Model file for the job. Use its own axes, mm. Round coordinates to 2 decimals unless told otherwise and drop trailing zeros. Order: outer loops, then holes, each group sorted by start corner. A loop starts at its lowest first (then second) coordinate and runs counter-clockwise, first axis right, second up. Notation, with made-up numbers: (53.5, 16.5) - (71.5, 16.5) arc R23 cw to (71.5, 40.5) - close; hole circle Ø4 at (-4.5, 36.5). An arc over 180 degrees is marked (long way). Use one line per item in the form item = value.
from build123d import *

# Parameters (mm, degrees)
SKETCH1_W               = 210
SKETCH1_H               = 110
TOP_DEPTH               = 5
SKETCH2_W               = 200
SKETCH2_H               = 100
BOTTOM_DEPTH            = 6
HOLE_REACH              = 120.684
SKETCH4_R               = 1.5
HOLE_PATTERN_COUNT      = 2
HOLE_PATTERN_PITCH      = 105
HOLE_PATTERN_COUNT_DIR2 = 2
HOLE_PATTERN_PITCH_DIR2 = 205


with BuildPart() as part:
    # Sketch1 → Top (new body)
    with BuildSketch(Plane(origin=(0, 0, 0), x_dir=(1, 0, 0), z_dir=(0, 1, 0))):
        Rectangle(SKETCH1_W, SKETCH1_H)
    extrude(amount=TOP_DEPTH)

    # Sketch2 → Bottom (add)
    with BuildSketch(Plane(origin=(0, 5, 0), x_dir=(1, 0, 0), z_dir=(0, 1, 0))):
        Rectangle(SKETCH2_W, SKETCH2_H)
    extrude(amount=BOTTOM_DEPTH)

    # Sketch4 → Hole (cut, up to next)
    with BuildSketch(Plane(origin=(0, 5, 0), x_dir=(1, 0, 0), z_dir=(0, 1, 0)), mode=Mode.PRIVATE) as hole_sk1:
        with Locations(Location((-102.5, -52.5, 0), (0, 0, 270))):
            Circle(SKETCH4_R)
    hole_tool1 = extrude(hole_sk1.sketch, amount=-HOLE_REACH, mode=Mode.PRIVATE) & part.part
    hole = hole_tool1.solids().sort_by_distance((-102.5, 5, 52.5))[0]
    add(hole, mode=Mode.SUBTRACT)

    # Hole-Pattern: Hole 2 × 2
    with Locations(*[(j * HOLE_PATTERN_PITCH_DIR2, 0, -i * HOLE_PATTERN_PITCH) for i in range(HOLE_PATTERN_COUNT) for j in range(HOLE_PATTERN_COUNT_DIR2) if (i, j) != (0, 0)]):
        add(hole, mode=Mode.SUBTRACT)


solid = part.part
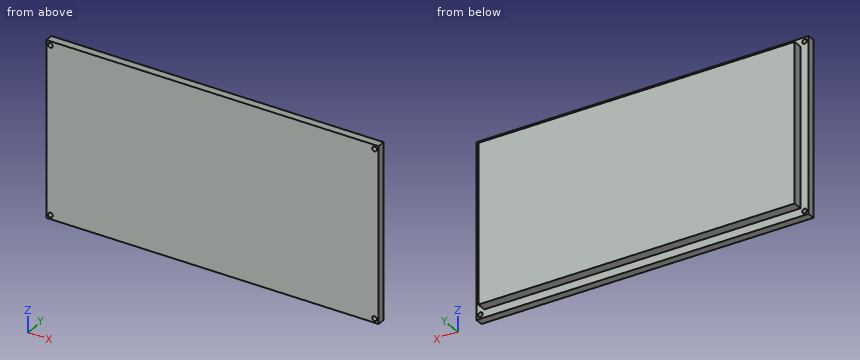
(1) Slice it at A-A on x = 16.5. Give the cut face in (y, z).
Report:
outline = (0, -55) - (5, -55) - (5, -50) - (11, -50) - (11, 50) - (5, 50) - (5, 55) - (0, 55) - close
(2) Pin check, flat tips, straight feed: pin 1 (1.8 mm diameter, centred on y = 8.5, z = 16, fed in from +X); pin 2 (1.8 mm diameter, centred on x = -102.5, z = 52.5, fed in from -Y); pin 3 (3.5 mm diameter, centred on x = -102.5, z = -52.5, fed in from +Y); pin 4 (5 mm diameter, centred on x = 40.5, y = 9, fed in from +Z). Stop position of each tip, or through.
Report:
pin_1 = 100
pin_2 = through
pin_3 = 5
pin_4 = 50
(3) Probe probe 1 along X at (y, z) = (1.5, -52.5); probe 2 along Z at (x, y) = (-102.5, 3.95); probe 3 along X at (y, z) = (10, 15). List the from-to ranges inside material, lowest first. Write a range as [from, to].
Report:
probe_1 = [-105, -104], [-101, 101], [104, 105]
probe_2 = [-55, -54], [-51, 51], [54, 55]
probe_3 = [-100, 100]
(4) Slice it at B-B on z = -35. Give the cut face in (x, y), then the cut area to 3 significant figures.
Report:
outline = (-105, 0) - (105, 0) - (105, 5) - (100, 5) - (100, 11) - (-100, 11) - (-100, 5) - (-105, 5) - close
area = 2,250 mm2
